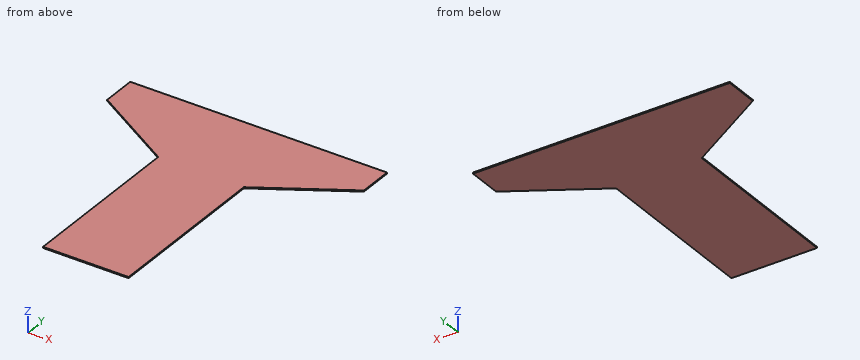
from build123d import *

# Parameters (mm, degrees)
BOSS_EXTRUDE1_DEPTH = 0.666666667
SCALE1_SCALE        = 3


with BuildPart() as part:
    # Sketch1 → Boss-Extrude1 (new body)
    with BuildSketch(Plane.XY):
        Polygon((75, 0), (-75, 0), (-75, -20), (-25, -50), (-25, -149.999999898), (25, -149.999999898), (25, -50), (75, -20), align=None)
    extrude(amount=BOSS_EXTRUDE1_DEPTH)


with BuildPart() as part_1:
    # Scale1: scaled about (0, -57.045454502, 0.333333333)
    add(part.part.scale(SCALE1_SCALE).moved(Location((0, 114.090909004, -0.666666666))))


solid = part_1.part
Here's how the part is built. I have some questions about the finished solid (model axes, mm). Coordinates: 2 decimals unless noted, no trailing zeros. Write each loop counter-clockwise with the first axis right and the second up, starting at its lowest first coordinate (ties: lowest second). Pieces come first, ordered by that corner, then holes.
Item 1: I want a section at B-B on y = -2.5. Write out the boundary of the cut face in (x, z).
Item 2: If I drill on line 1 (X direction, y = -120.5, z = 0.75); line 2 (Y direction, x = -76, z = 0.4); line 3 (Y direction, x = 87.5, z = 0.7), over which ranges is the centre line in solid material (lowest first)?
Item 3: I want a section at C-C on x = -186.5. Write out the boundary of the cut face in (y, z).
Item 4: I want a section at A-A on z = 0.6. Write out the boundary of the cut face in (x, y).
Item 5: Will this pin go through, and if not, where does the flat tip stop? pin 1 (0.6 mm diameter, centred on y = -235.5, z = 0.5, fed in from +X).
Findings below:
1. outline: (-130.68, -0.67) - (130.68, -0.67) - (130.68, 1.33) - (-130.68, 1.33) - close
2. line 1: x = -75 to 75
2. line 2: y = -35.31 to 114.09
2. line 3: y = -28.41 to 114.09
3. outline: (30.99, -0.67) - (114.09, -0.67) - (114.09, 1.33) - (30.99, 1.33) - close
4. outline: (-225, 54.09) - (-75, -35.91) - (-75, -335.91) - (75, -335.91) - (75, -35.91) - (225, 54.09) - (225, 114.09) - (-225, 114.09) - close
5. pin 1: stops at x = 75
